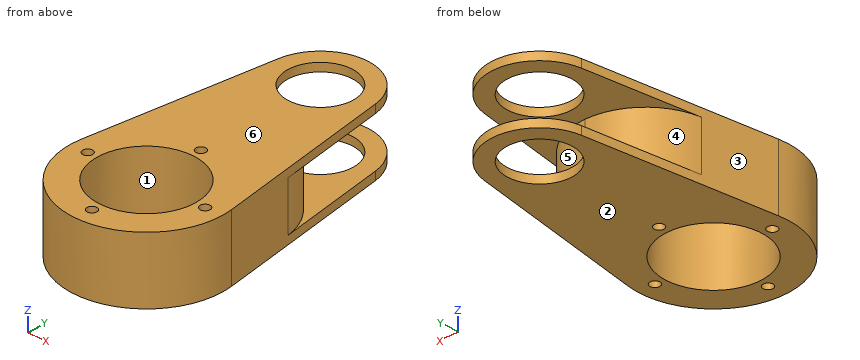
from build123d import *

# Parameters (mm, degrees)
CROQUIS1_R                 = 15
CROQUIS1_R_2               = 1.5
CROQUIS1_R_3               = 10
SALIENTE_EXTRUIR1_DEPTH    = 10
CORTAR_EXTRUIR2_DEPTH      = 24.25
CORTAR_EXTRUIR2_DEPTH_BACK = 24.25
REDONDEO3_R                = 20


with BuildPart() as part:
    # Croquis1 → Saliente-Extruir1 (new body, symmetric)
    with BuildSketch(Plane.XY):
        with BuildLine():
            Line((-23.009443154, 3.997898972), (-14.844802035, 60.31420332))
            ThreePointArc((-14.844802035, 60.31420332), (0, 73.162029407), (14.844802035, 60.31420332))
            Line((14.844802035, 60.31420332), (23.009443154, 3.997898972))
            ThreePointArc((23.009443154, 3.997898972), (0, -22.587970593), (-23.009443154, 3.997898972))
        make_face()
        with Locations((0, 0.662029407)):
            Circle(CROQUIS1_R, mode=Mode.SUBTRACT)
        with Locations((0, 18.662029407)):
            Circle(CROQUIS1_R_2, mode=Mode.SUBTRACT)
        with Locations((18, 0.662029407)):
            Circle(CROQUIS1_R_2, mode=Mode.SUBTRACT)
        with Locations((0, -17.337970593)):
            Circle(CROQUIS1_R_2, mode=Mode.SUBTRACT)
        with Locations((-18, 0.662029407)):
            Circle(CROQUIS1_R_2, mode=Mode.SUBTRACT)
        with Locations((0, 58.162029407)):
            Circle(CROQUIS1_R_3, mode=Mode.SUBTRACT)
    extrude(amount=SALIENTE_EXTRUIR1_DEPTH, both=True)

    # Croquis3 → Cortar-Extruir2 (cut, two sides)
    with BuildSketch(Plane(origin=(0, 0, 0), x_dir=(0, 0, -1), z_dir=(1, 0, 0))) as cortar_extruir2_sk:
        Polygon((0, 73.162029407), (7.5, 73.162029407), (7.5, 43.162029407), (-7.5, 43.162029407), (-7.5, 73.162029407), align=None)
    extrude(amount=CORTAR_EXTRUIR2_DEPTH, mode=Mode.SUBTRACT)
    extrude(cortar_extruir2_sk.sketch, amount=-CORTAR_EXTRUIR2_DEPTH_BACK, mode=Mode.SUBTRACT)

    # Redondeo3
    redondeo3_edges = [part.edges().sort_by_distance(p)[0] for p in [
        (-17.331494761, 43.162029407, 0),
        (17.331494761, 43.162029407, 0),
    ]]
    fillet(redondeo3_edges, radius=REDONDEO3_R)


solid = part.part
Work out the finished part from the listing and answer in its coordinate system (mm). Face numbers are marked on the shaded views. A direction names the side the tool comes from. Coordinates: 2 decimals unless noted, no trailing zeros. Write each loop counter-clockwise with the first axis right and the second up, starting at its lowest first coordinate (ties: lowest second). Pieces come first, ordered by that corner, then holes. Notation, with made-up numbers: (30, 47) - (65, 47) arc R35 ccw to (65, 83) - close; hole circle Ø6 at (36, 45). An arc over 180 degrees is marked (long way). One line per question, with ' | ' between items.
1) Flat-ended cylindrical pins translate along their axes: P1, Ø2, axis at x = -10.5, z = -7, coming from the +Y side; P2, Ø6, axis at y = 27.5, z = 0, coming from the -X side; P3, Ø4, axis at x = -18, z = -4, coming from the +Y side. Find the tip coordinate at first contact, or state that the pin passes through.
Checks:
P1: y = 69.66 | P2: x = -20.04 | P3: y = 35.19
2) Find section B-B, the plane x = 9. Determine the outline of the cut face in (y, z).
Checks:
outline: (-20.78, -10) - (-11.34, -10) - (-11.34, 10) - (-20.78, 10) - close; (12.66, -10) - (53.8, -10) - (53.8, -7.5) - (41.03, -7.5) - (41.03, 7.5) - (53.8, 7.5) - (53.8, 10) - (12.66, 10) - close; (62.52, -10) - (70.16, -10) - (70.16, -7.5) - (62.52, -7.5) - close; (62.52, 7.5) - (70.16, 7.5) - (70.16, 10) - (62.52, 10) - close
3) Find section C-C, the plane z = -4.25. Determine the outline of the cut face in (x, y), and give its area (3 significant figures).
Checks:
outline: (-23.01, 4) arc R23.25 ccw (long way) to (23.01, 4) - (19.82, 26.03) arc R20 ccw to (0.02, 43.16) - (-0.02, 43.16) arc R20 ccw to (-19.82, 26.03) - close; hole circle Ø3 at (-18, 0.66); hole circle Ø30 at (0, 0.66); hole circle Ø3 at (0, -17.34); hole circle Ø3 at (0, 18.66); hole circle Ø3 at (18, 0.66) | area: 1,730 mm2
4) Consider probe 1 along Y at (x, z) = (0, 9.1); probe 2 along Z at (x, y) = (15, 56); probe 3 along Y at (x, z) = (0, -2.5). Determine where each line is inside the solid, lowest interval first. Write a range as [from, to].
Checks:
probe 1: [-22.59, -18.84], [-15.84, -14.34], [15.66, 17.16], [20.16, 48.16], [68.16, 73.16] | probe 2: [-10, -7.5], [7.5, 10] | probe 3: [-22.59, -18.84], [-15.84, -14.34], [15.66, 17.16], [20.16, 43.16]
5) The mould has two halves that part along Y. Classify the marked faces 1, 2 and 3: +Y half, -Y half, draft (parallel to the pull), parting line (faces both ways), or undercut.
Checks:
face 1: undercut | face 2: draft | face 3: +Y half
6) Find section A-A, the plane y = 50.5. Determine the outline of the cut face in (x, z).
Checks:
outline: (-16.27, -10) - (-6.43, -10) - (-6.43, -7.5) - (-16.27, -7.5) - close; (-16.27, 7.5) - (-6.43, 7.5) - (-6.43, 10) - (-16.27, 10) - close; (6.43, -10) - (16.27, -10) - (16.27, -7.5) - (6.43, -7.5) - close; (6.43, 7.5) - (16.27, 7.5) - (16.27, 10) - (6.43, 10) - close
7) Find section D-D, the plane x = -11.5. Determine the outline of the cut face in (y, z).
Checks:
outline: (-19.54, -10) - (-8.97, -10) - (-8.97, 10) - (-19.54, 10) - close; (10.29, -10) - (67.79, -10) - (67.79, -7.5) - (39.54, -7.5) - (39.54, 7.5) - (67.79, 7.5) - (67.79, 10) - (10.29, 10) - close
8) For the marked faces 4, 5 and 6, determine the directions among +Z, -Z, +X, -X, +Y, -Y from which every point of the face is accessible in a straight line to the end or side of a thin tool.
Checks:
face 4: -X, +Y | face 5: +X, +Y | face 6: +Z, +X, -X, +Y, -Y
